from build123d import *

# Parameters (mm, degrees)
SKETCH1_W           = 3.17
SKETCH1_H           = 25
SKETCH1_W_2         = 3.175
BOSS_EXTRUDE1_DEPTH = 6.35


with BuildPart() as part:
    # Sketch1 → Boss-Extrude1 (new body)
    with BuildSketch(Plane.XY):
        Polygon((0, 0), (0, 403.175), (16.666666667, 403.175), (16.666666667, 409.425), (33.333333333, 409.425), (33.333333333, 403.175), (50, 403.175), (50, 0), (33.333333333, 0), (33.333333333, -12.7), (16.666666667, -12.7), (16.666666667, 0), align=None)
        with Locations((34.918333333, 137.5)):
            Rectangle(SKETCH1_W, SKETCH1_H, mode=Mode.SUBTRACT)
        with Locations((34.920833333, 37.5)):
            Rectangle(SKETCH1_W_2, SKETCH1_H, mode=Mode.SUBTRACT)
        with Locations((15.079166667, 37.5)):
            Rectangle(SKETCH1_W_2, SKETCH1_H, mode=Mode.SUBTRACT)
        with Locations((34.918333333, 87.5)):
            Rectangle(SKETCH1_W, SKETCH1_H, mode=Mode.SUBTRACT)
        with Locations((15.079166667, 87.5)):
            Rectangle(SKETCH1_W_2, SKETCH1_H, mode=Mode.SUBTRACT)
        with Locations((15.079166667, 137.5)):
            Rectangle(SKETCH1_W_2, SKETCH1_H, mode=Mode.SUBTRACT)
        with Locations((34.918333333, 187.5)):
            Rectangle(SKETCH1_W, SKETCH1_H, mode=Mode.SUBTRACT)
        with Locations((15.079166667, 187.5)):
            Rectangle(SKETCH1_W_2, SKETCH1_H, mode=Mode.SUBTRACT)
        with Locations((34.918333333, 237.5)):
            Rectangle(SKETCH1_W, SKETCH1_H, mode=Mode.SUBTRACT)
        with Locations((15.079166667, 237.5)):
            Rectangle(SKETCH1_W_2, SKETCH1_H, mode=Mode.SUBTRACT)
        with Locations((34.918333333, 287.5)):
            Rectangle(SKETCH1_W, SKETCH1_H, mode=Mode.SUBTRACT)
        with Locations((15.079166667, 287.5)):
            Rectangle(SKETCH1_W_2, SKETCH1_H, mode=Mode.SUBTRACT)
        with Locations((34.918333333, 337.5)):
            Rectangle(SKETCH1_W, SKETCH1_H, mode=Mode.SUBTRACT)
        with Locations((15.079166667, 337.5)):
            Rectangle(SKETCH1_W_2, SKETCH1_H, mode=Mode.SUBTRACT)
        with Locations((34.918333333, 387.5)):
            Rectangle(SKETCH1_W, SKETCH1_H, mode=Mode.SUBTRACT)
        with Locations((15.079166667, 387.5)):
            Rectangle(SKETCH1_W_2, SKETCH1_H, mode=Mode.SUBTRACT)
    extrude(amount=BOSS_EXTRUDE1_DEPTH)


solid = part.part
Geometry check sheet. Reference: the model listing, model coordinates, mm. Round coordinates to 2 decimals unless told otherwise and drop trailing zeros. Write each loop counter-clockwise with the first axis right and the second up, starting at its lowest first coordinate (ties: lowest second). Pieces come first, ordered by that corner, then holes. Notation, with made-up numbers: (24, 51) - (83, 51) arc R29 cw to (83, 79) - close; hole circle Ø8 at (78, 54.5). An arc over 180 degrees is marked (long way). One line per item, written item: value.
1. Depth check by flat-ended pin: pin 1 Ø1.6 at (x, z) = (16, 2.5) entering from +Y (3 decimals); pin 2 Ø1.6 at (x, z) = (14.5, 2.5) entering from -Y; pin 3 Ø1 at (x, z) = (35.5, 4) entering from +Y (3 decimals). Enter the tip coordinate at first touch or a pass-through.
The answers:
pin 1: stops at y = 409.425
pin 2: stops at y = 0
pin 3: stops at y = 403.175
2. Cross-section at A-A on y = 337. Record the boundary of the cut face in (x, z), and give its area (3 significant figures).
The answers:
outline: (0, 0) - (13.49, 0) - (13.49, 6.35) - (0, 6.35) - close; (16.67, 0) - (33.33, 0) - (33.33, 6.35) - (16.67, 6.35) - close; (36.5, 0) - (50, 0) - (50, 6.35) - (36.5, 6.35) - close
area: 277 mm^2
3. Cross-section at B-B on z = 2.75. Give the number of separate pieces and of enclosed holes in the cut face, and give its area (3 significant figures).
The answers:
separate pieces: 1
enclosed holes: 16
area: 19,200 mm^2
4. Cross-section at C-C on x = 6.5. Record the boundary of the cut face in (y, z) (3 decimals), and give its area (3 significant figures).
The answers:
outline: (0, 0) - (403.175, 0) - (403.175, 6.35) - (0, 6.35) - close
area: 2,560 mm^2
5. Scan lines: L1, parallel to X at y = 147, z = 1.5; L2, parallel to Y at x = 9, z = 5.5 (3 decimals). Record each from-to range of solid material in increasing order.
The answers:
L1: x = 0 to 13.49, 16.67 to 33.33, 36.5 to 50
L2: y = 0 to 403.175
